Build history of the part. All positions in model axes, mm. Round coordinates to 2 decimals unless told otherwise and drop trailing zeros. Order: outer loops, then holes, each group sorted by start corner. A loop starts at its lowest first (then second) coordinate and runs counter-clockwise, first axis right, second up. Notation, with made-up numbers: (28.5, 11) -> (63.5, 11) arc R34 ccw to (63.5, 49) -> close; hole circle Ø6 at (73, 28). An arc over 180 degrees is marked (long way). Write item = value, one per line.
from build123d import *

# Parameters (mm, degrees)
SKETCH1_R            = 3
BOSS_EXTRUDE1_DEPTH  = 15.275
M3_CLEARANCE_HOLE1_D = 3.2
CHAMFER1_SIZE        = 0.25


with BuildPart() as part:
    # Sketch1 → Boss-Extrude1 (new body)
    with BuildSketch(Plane(origin=(0, 0, 0), x_dir=(1, 0, 0), z_dir=(0, 1, 0))):
        with Locations(Location((0, 0, 0), (0, 0, 270))):
            Circle(SKETCH1_R)
    extrude(amount=BOSS_EXTRUDE1_DEPTH)

    # M3 Clearance Hole1 (through all)
    with Locations(Plane(origin=(0, 15.275, 0), x_dir=(1, 0, 0), z_dir=(0, 1, 0))):
        with Locations((0, 0)):
            Hole(M3_CLEARANCE_HOLE1_D / 2)

    # Chamfer1
    chamfer1_edges = [part.edges().sort_by_distance(p)[0] for p in [
        (1.6, 15.275, 0),
        (1.6, 0, 0),
    ]]
    chamfer(chamfer1_edges, length=CHAMFER1_SIZE)


solid = part.part
Q1. Cut at A-A, the plane x = 0. List the corners of the cut face in (y, z) (3 decimals), and give its area (3 significant figures).
Check values:
outline = (0, -3) -> (15.275, -3) -> (15.275, -1.85) -> (15.025, -1.6) -> (0.25, -1.6) -> (0, -1.85) -> close; (0, 1.85) -> (0.25, 1.6) -> (15.025, 1.6) -> (15.275, 1.85) -> (15.275, 3) -> (0, 3) -> close
area = 42.6 mm²
Q2. Probe probe 1 along X at (y, z) = (8.25, 0); probe 2 along X at (y, z) = (14, 1). List the from-to ranges inside material, lowest first.
Check values:
probe_1 = -3 to -1.6, 1.6 to 3
probe_2 = -2.83 to -1.25, 1.25 to 2.83
Q3. Flat gauge pins, fed straight in: pin 1 (2 mm diameter, centred on y = 7.5, z = 2, fed in from -X); pin 2 (3.5 mm diameter, centred on x = 0, z = 0, fed in from +Y) (3 decimals); pin 3 (2 mm diameter, centred on x = 2, y = 3.5, fed in from -Z). Where does each tip first touch, or does it go through?
Check values:
pin_1 = -2.83
pin_2 = 15.175
pin_3 = -2.83
Q4. Cut at D-D, the plane z = 2.5. List the corners of the cut face in (x, y) (3 decimals), and give its area (3 significant figures).
Check values:
outline = (-1.658, 0) -> (1.658, 0) -> (1.658, 15.275) -> (-1.658, 15.275) -> close
area = 50.7 mm²
Q5. Cut at B-B, the plane z = 0. List the corners of the cut face in (x, y) (3 decimals), and give its area (3 significant figures).
Check values:
outline = (-3, 0) -> (-1.85, 0) -> (-1.6, 0.25) -> (-1.6, 15.025) -> (-1.85, 15.275) -> (-3, 15.275) -> close; (1.6, 0.25) -> (1.85, 0) -> (3, 0) -> (3, 15.275) -> (1.85, 15.275) -> (1.6, 15.025) -> close
area = 42.6 mm²
Q6. Mould opens along X. For faces 1 (the face through (1.27, 7.53, 0.97)), 2 (the face through (-2, 0, 1)), 3 (the face through (0.9, 7.53, 2.86)) say: released by +X, released by -X, zero draft, split by the parting line, or undercut.
Check values:
face_1 = undercut
face_2 = zero draft
face_3 = split by the parting line
Q7. Cut at C-C, the plane y = 9. List the corners of the cut face in (x, z), and give its area (3 significant figures).
Check values:
outline = circle Ø6 at (0, 0); hole circle Ø3.2 at (0, 0)
area = 20.2 mm²
